The listing builds one solid part. Answer for the finished solid, in the listing's coordinates (mm). A direction names the side the tool comes from. Coordinates: 2 decimals unless noted, no trailing zeros. Order: outer loops, then holes, each group sorted by start corner. A loop starts at its lowest first (then second) coordinate and runs counter-clockwise, first axis right, second up. Notation, with made-up numbers: (-9, -2.75) -> (14, -2.75) arc R21 ccw to (14, 10.25) -> close; hole circle Ø10 at (35.5, 35). An arc over 180 degrees is marked (long way). Return JSON: item names as keys, results as strings.
from build123d import *

# Parameters (mm, degrees)
SKETCH1_R           = 111.125
SKETCH1_R_2         = 3.96875
SKETCH1_R_3         = 8
SKETCH1_W           = 14
SKETCH1_H           = 14
SKETCH1_W_2         = 23
SKETCH1_H_2         = 10.5
BOSS_EXTRUDE1_DEPTH = 1.5875


with BuildPart() as part:
    # Sketch1 → Boss-Extrude1 (new body)
    with BuildSketch(Plane(origin=(0, 0, 0), x_dir=(1, 0, 0), z_dir=(0, 1, 0))):
        Circle(SKETCH1_R)
        with Locations((0, 22.225)):
            Circle(SKETCH1_R_2, mode=Mode.SUBTRACT)
        with Locations((19.247414599, -11.1125)):
            Circle(SKETCH1_R_2, mode=Mode.SUBTRACT)
        with Locations((-19.247414599, -11.1125)):
            Circle(SKETCH1_R_2, mode=Mode.SUBTRACT)
        with Locations((-48, -12.5)):
            Circle(SKETCH1_R_3, mode=Mode.SUBTRACT)
        with Locations((-69.650635095, 0)):
            Circle(SKETCH1_R_3, mode=Mode.SUBTRACT)
        with Locations((-48, 12.5)):
            Circle(SKETCH1_R_3, mode=Mode.SUBTRACT)
        with Locations((48, 12.5)):
            Rectangle(SKETCH1_W, SKETCH1_H, mode=Mode.SUBTRACT)
        with Locations((0, -37.246432928)):
            Rectangle(SKETCH1_W_2, SKETCH1_H_2, mode=Mode.SUBTRACT)
        with Locations((48, -12.5)):
            Rectangle(SKETCH1_W, SKETCH1_H, mode=Mode.SUBTRACT)
        with BuildLine():
            ThreePointArc((86.299834064, 32.095860566), (0, 92.075), (-86.299834064, 32.095860566))
            ThreePointArc((-86.299834064, 32.095860566), (-84.832280885, 25.386264259), (-78.118809332, 23.936541993))
            ThreePointArc((-78.118809332, 23.936541993), (0, 38.1), (78.118809332, 23.936541993))
            ThreePointArc((78.118809332, 23.936541993), (84.832280885, 25.386264259), (86.299834064, 32.095860566))
        make_face(mode=Mode.SUBTRACT)
        with BuildLine():
            ThreePointArc((-80.484779709, -20.088608264), (-40.736920582, -40.736920582), (-20.088608264, -80.484779709))
            ThreePointArc((-20.088608264, -80.484779709), (-22.177824514, -86.368987271), (-28.295419505, -87.619489042))
            ThreePointArc((-28.295419505, -87.619489042), (-65.106856878, -65.106856878), (-87.619489042, -28.295419505))
            ThreePointArc((-87.619489042, -28.295419505), (-86.368987271, -22.177824514), (-80.484779709, -20.088608264))
        make_face(mode=Mode.SUBTRACT)
        with BuildLine():
            ThreePointArc((20.088608264, -80.484779709), (40.736920582, -40.736920582), (80.484779709, -20.088608264))
            ThreePointArc((80.484779709, -20.088608264), (86.368987271, -22.177824514), (87.619489042, -28.295419505))
            ThreePointArc((87.619489042, -28.295419505), (65.106856878, -65.106856878), (28.295419505, -87.619489042))
            ThreePointArc((28.295419505, -87.619489042), (22.177824514, -86.368987271), (20.088608264, -80.484779709))
        make_face(mode=Mode.SUBTRACT)
    extrude(amount=BOSS_EXTRUDE1_DEPTH)


solid = part.part
1. The part is cut by section D-D on x = -48. Give the vertices of the cut face in (y, z), and give its area (3 significant figures).
Answer block:
{"outline": "(0, -100.22) -> (1.59, -100.22) -> (1.59, -78.57) -> (0, -78.57) -> close; (0, -32.86) -> (1.59, -32.86) -> (1.59, -20.5) -> (0, -20.5) -> close; (0, -4.5) -> (1.59, -4.5) -> (1.59, 4.5) -> (0, 4.5) -> close; (0, 20.5) -> (1.59, 20.5) -> (1.59, 34.36) -> (0, 34.36) -> close; (0, 78.57) -> (1.59, 78.57) -> (1.59, 100.22) -> (0, 100.22) -> close", "area": "125 mm2"}
2. The part is cut by section A-A on z = 0. Give the vertices of the cut face in (x, y) (1 decimal), and give its area (3 significant figures).
Answer block:
{"outline": "(-111.1, 0) -> (-77.7, 0) -> (-77.7, 1.6) -> (-111.1, 1.6) -> close; (-61.7, 0) -> (111.1, 0) -> (111.1, 1.6) -> (-61.7, 1.6) -> close", "area": "327 mm2"}
3. The part is cut by section B-B on x = 0. Give the vertices of the cut face in (y, z) (1 decimal), and give its area (3 significant figures).
Answer block:
{"outline": "(0, -111.1) -> (1.6, -111.1) -> (1.6, -92.1) -> (0, -92.1) -> close; (0, -38.1) -> (1.6, -38.1) -> (1.6, -26.2) -> (0, -26.2) -> close; (0, -18.3) -> (1.6, -18.3) -> (1.6, 32) -> (0, 32) -> close; (0, 42.5) -> (1.6, 42.5) -> (1.6, 111.1) -> (0, 111.1) -> close", "area": "238 mm2"}
4. Consider line 1 (X direction, y = 0.45, z = 0) (3 decimals); line 2 (X direction, y = 1.3, z = -14.5); line 3 (X direction, y = 1.25, z = -12.5). Determine where each line is inside the solid, lowest interval first. Write a range as from..to.
Answer block:
{"line 1": "x = -111.125..-77.651, -61.651..111.125", "line 2": "x = -110.17..-55.75, -40.25..41, 55..110.17", "line 3": "x = -110.42..-56, -40..41, 55..110.42"}
5. Determine the mould class of faces 1 (the face through (-2, 0, -2)), 2 (the face through (84.76, 0.783, -25.315)) for opening direction Z: pulls with the +Z half, pulls with the -Z half, needs draft (parallel to the pull), parting line crosses it, or undercut.
Answer block:
{"face 1": "needs draft", "face 2": "undercut"}
6. The part is cut by section C-C on y = 1.05. Give the number of separate pieces and of enclosed holes in the cut face, and give its area (3 significant figures).
Answer block:
{"separate pieces": "1", "enclosed holes": "12", "area": "25,300 mm2"}
7. For faces 3 (the face through (-1.117, 0.783, -38.097)), 4 (the face through (-2, 1.588, -2)), determine the directions among +Z, -Z, +X, -X, +Y, -Y from which every point of the face is accessible in a straight line to the end or side of a thin tool.
Answer block:
{"face 3": "+Y, -Y", "face 4": "+Z, -Z, +X, -X, +Y"}
8. Each of these flat-tipped pins is pushed along its axis until it touches: pin 1 Ø0.8 at (y, z) = (1, -9.5) entering from -X; pin 2 Ø0.5 at (x, y) = (50.5, 1) entering from +Z; pin 3 Ø0.8 at (x, y) = (45.5, 0.5) entering from -Z; pin 4 Ø18.5 at (x, z) = (-69.65, 0) entering from -Y. Where does it stop, or does it pass through?
Answer block:
{"pin 1": "stops at x = -110.75", "pin 2": "stops at z = 99.11", "pin 3": "stops at z = -101.56", "pin 4": "stops at y = 0"}
